from build123d import *

# Parameters (mm, degrees)
F0_W           = 635
F0_H           = 635
F1_DEPTH       = 25.4
F9_DEPTH       = 12.7
F2_R           = 127
F3_W           = 457.2
F3_H           = 457.2
F4_DEPTH       = 3.175
F5_R           = 127
F7_D           = 3.175
F7_DEPTH       = 63.5
F7_CBORE_D     = 12.7
F7_CBORE_DEPTH = 3.175


with BuildPart() as f1:
    # F0 (on Top) → F1 (new body)
    with BuildSketch(Plane.XY):
        Rectangle(F0_W, F0_H)
    extrude(amount=F1_DEPTH)

    # F8 (on face) → F9 (cut)
    with BuildSketch(Plane.XY.offset(25.4)):
        Polygon((12.7, 12.7), (12.7, 165.1), (-12.7, 165.1), (-12.7, 12.7), (-165.1, 12.7), (-165.1, -12.7), (-12.7, -12.7), (-12.7, -165.1), (12.7, -165.1), (12.7, -12.7), (165.1, -12.7), (165.1, 12.7), align=None)
    extrude(amount=-F9_DEPTH, mode=Mode.SUBTRACT)

    # F2
    f2_edges = [f1.edges().sort_by_distance(p)[0] for p in [
        (-317.5, -317.5, 12.7),
        (317.5, -317.5, 12.7),
        (317.5, 317.5, 12.7),
        (-317.5, 317.5, 12.7),
    ]]
    fillet(f2_edges, radius=F2_R)

    # F3 (on face) → F4 (cut)
    with BuildSketch(Plane(origin=(0, 0, 0), x_dir=(1, 0, 0), z_dir=(0, 0, -1))):
        Rectangle(F3_W, F3_H)
    extrude(amount=-F4_DEPTH, mode=Mode.SUBTRACT)

    # F5
    f5_edges = [f1.edges().sort_by_distance(p)[0] for p in [
        (-228.6, -228.6, 1.5875),
        (228.6, -228.6, 1.5875),
        (228.6, 228.6, 1.5875),
        (-228.6, 228.6, 1.5875),
    ]]
    fillet(f5_edges, radius=F5_R)

    # F7
    with Locations(Plane(origin=(0, 0, 3.175), x_dir=(1, 0, 0), z_dir=(0, 0, -1))):
        with Locations((-127, 0), (127, 0), (0, 127), (0, -127)):
            CounterBoreHole(F7_D / 2, F7_CBORE_D / 2, F7_CBORE_DEPTH, depth=F7_DEPTH)


solid = f1.part
For this review, take the finished solid that the model builds, in its own axes (mm). A direction names the side the tool comes from. Give positions to 0.01 mm unless a question says otherwise; leave off trailing zeros. Loops run counter-clockwise (first coordinate to the right, second up) from the corner with the lowest first, then second, coordinate; pieces in that order, holes last. Notation, with made-up numbers: M 23,7.25 L 43,7.25 A16 cw 43,22.25 Z; hole C 58,-23.5 d10. An arc over 180 degrees is marked long. Put each result on its own line as item: value. Start each with the question number.
(1) For pin 1 (10 mm diameter, centred on x = -148.5, y = -13, fed in from -Z) (3 decimals); pin 2 (1 mm diameter, centred on y = 239, z = 5, fed in from +X); pin 3 (1.5 mm diameter, centred on y = -231.5, z = 10.5, fed in from +X), all flat-tipped, find the tip position at first contact; note any pin that passes through.
(2) Wall thickness on L1, parallel to Y at x = 0, z = 5; L2, parallel to X at y = -118, z = 24.5; L3, parallel to X at y = 127, z = 9: over which ranges is each line inside the solid? List them lowest first.
(3) Machinability: for faces 4 (the cylindrical face through (279.31, 281.285, 12.878)), 5 (the flat face through (-3, -3, 3.175)), which of the approach directions +Z, -Z, +X, -X, +Y, -Y give a long, thin tool a straight path to every point of the face, cutting with its end or side? Answer none if there is none.
(4) The part is to be moulded in two halves that separate along Y. For faces 1 (the flat face through (-3, -317.5, 13)), 2 (the flat face through (66, -66, 25.4)), 3 (the cylindrical face through (192.385, 190.41, 1.61)), say which applies: +Y half, -Y half, draft (parallel to the pull), parting line (faces both ways), or undercut.
(5) Add section A-A, the plane y = -61.5. Write out the cut boundary in (x, z) (3 decimals), then the cut area to 3 significant figures.
(6) Add section B-B, the plane y = -148.5. Write out the cut boundary in (x, z) (3 decimals).
(7) Add section C-C, the plane y = -213. Write out the cut boundary in (x, z) (3 decimals), then the cut area to 3 significant figures.
Result:
1. pin 1: stops at z = 3.175
1. pin 2: stops at x = 308.08
1. pin 3: stops at x = 310.95
2. L1: y = -317.5 to -133.35, -120.65 to 120.65, 133.35 to 317.5
2. L2: x = -317.5 to -12.7, 12.7 to 317.5
2. L3: x = -317.5 to -1.59, 1.59 to 317.5
3. face 4: +Z, -Z, +X, +Y
3. face 5: -Z
4. face 1: -Y half
4. face 2: draft
4. face 3: undercut
5. outline: M -317.5,0 L -228.6,0 L -228.6,3.175 L 228.6,3.175 L 228.6,0 L 317.5,0 L 317.5,25.4 L 12.7,25.4 L 12.7,12.7 L -12.7,12.7 L -12.7,25.4 L -317.5,25.4 Z
5. area: 14,400 mm^2
6. outline: M -317.5,0 L -219.623,0 L -219.623,3.175 L 219.623,3.175 L 219.623,0 L 317.5,0 L 317.5,25.4 L 12.7,25.4 L 12.7,12.7 L -12.7,12.7 L -12.7,25.4 L -317.5,25.4 Z
7. outline: M -315.491,0 L -162.584,0 L -162.584,3.175 L 162.584,3.175 L 162.584,0 L 315.491,0 L 315.491,25.4 L -315.491,25.4 Z
7. area: 15,000 mm^2
